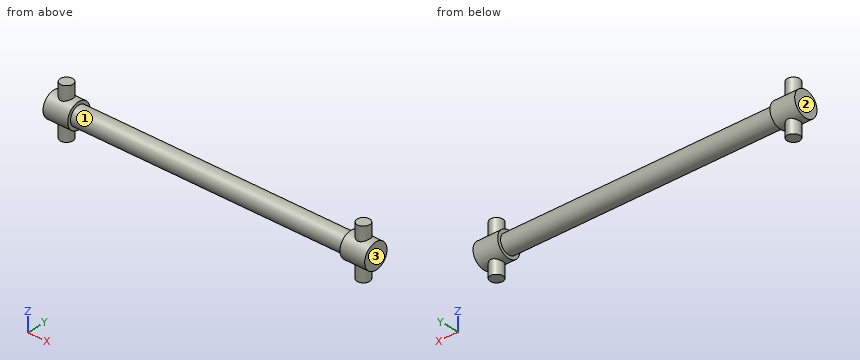
```python
from build123d import *

# Parameters (mm, degrees)
SKETCH1_R                = 1.5
BOSS_EXTRUDE1_DEPTH      = 52
SKETCH2_R                = 2
BOSS_EXTRUDE2_DEPTH      = 4
BOSS_EXTRUDE3_START      = -4
SKETCH3_R                = 2
BOSS_EXTRUDE3_DEPTH      = 4
BOSS_EXTRUDE4_DEPTH      = 2
BOSS_EXTRUDE4_DEPTH_BACK = 6
SKETCH4_R                = 1


with BuildPart() as part:
    # Sketch1 → Boss-Extrude1 (new body)
    with BuildSketch(Plane(origin=(0, 0, 0), x_dir=(0, 0, -1), z_dir=(1, 0, 0))):
        with Locations(Location((0, 0, 0), (0, 0, 180))):
            Circle(SKETCH1_R)
    extrude(amount=BOSS_EXTRUDE1_DEPTH)

    # Sketch2 → Boss-Extrude2 (add)
    with BuildSketch(Plane(origin=(52, 0, 0), x_dir=(0, 0, -1), z_dir=(1, 0, 0))):
        Circle(SKETCH2_R)
    extrude(amount=-BOSS_EXTRUDE2_DEPTH)

    # Sketch3 → Boss-Extrude3 (add)
    with BuildSketch(Plane.ZY.offset(BOSS_EXTRUDE3_START)):
        with Locations(Location((0, 0, 0), (0, 0, 180))):
            Circle(SKETCH3_R)
    extrude(amount=BOSS_EXTRUDE3_DEPTH)

    # Sketch4 → Boss-Extrude4 (add, two sides: drawn at the far end of the back side and taken through both)
    with BuildSketch(Plane.XY.offset(2).offset(-BOSS_EXTRUDE4_DEPTH_BACK)):
        with Locations((50, 0)):
            Circle(SKETCH4_R)
        with Locations((2, 0)):
            Circle(SKETCH4_R)
    extrude(amount=BOSS_EXTRUDE4_DEPTH + BOSS_EXTRUDE4_DEPTH_BACK)


solid = part.part
```
Read the model definition and answer for the solid it produces. Units are mm, in the model's axes. Face numbers are marked on the shaded views. Give positions to 0.01 mm unless a question says otherwise; leave off trailing zeros. Write each loop counter-clockwise with the first axis right and the second up, starting at its lowest first coordinate (ties: lowest second). Pieces come first, ordered by that corner, then holes. Notation, with made-up numbers: M 25,54.5 L 50,54.5 A23 cw 50,67.5 Z; hole C 26.25,43 d9. An arc over 180 degrees is marked long. Put each result on its own line as item: value. Start each with the question number.
1. The part is cut by section C-C, the plane z = 3. Give the vertices of the cut face in (x, y), and give its area (3 significant figures).
2. For a pull along X with two mould halves and no side action, classify the marked faces 1, 2 and 3 as released by +X, released by -X, zero draft, split by the parting line, or undercut.
3. The part is cut by section D-D, the plane x = 44. Give the vertices of the cut face in (y, z), and give its area (3 significant figures).
4. The part is cut by section A-A, the plane x = 50. Give the vertices of the cut face in (y, z), and give its area (3 significant figures).
5. Each of these flat-tipped pins is pushed along its axis until it touches: pin 1 Ø1 at (x, y) = (20, -1) entering from -Z; pin 2 Ø1 at (y, z) = (-1, 3) entering from -X. Where does it stop, or does it pass through?
6. The part is cut by section B-B, the plane z = 0. Give the vertices of the cut face in (x, y), and give its area (3 significant figures).
7. Consider line 1 along X through (y, z) = (0.75, 1.75); line 2 along Z through (x, y) = (7.5, 0.1); line 3 along X through (y, z) = (0.35, 3.5). Determine where each line is inside the solid, lowest interval first.
Final values:
1. outline: C 2,0 d2; C 50,0 d2
1. area: 6.28 mm²
2. face 1: undercut
2. face 2: released by -X
2. face 3: released by +X
3. outline: C 0,0 d3
3. area: 7.07 mm²
4. outline: M -1,-4 L 1,-4 L 1,-1.73 A2 ccw 1,1.73 L 1,4 L -1,4 L -1,1.73 A2 ccw -1,-1.73 Z
4. area: 20.9 mm²
5. pin 1: stops at z = -1.41
5. pin 2: stops at x = 1.13
6. outline: M 0,-2 L 4,-2 L 4,-1.5 L 48,-1.5 L 48,-2 L 52,-2 L 52,2 L 48,2 L 48,1.5 L 4,1.5 L 4,2 L 0,2 Z
6. area: 164 mm²
7. line 1: x = 0 to 4, 48 to 52
7. line 2: z = -1.5 to 1.5
7. line 3: x = 1.06 to 2.94, 49.06 to 50.94
